Design review of the part built by this model. Coordinates are the model's own, in mm. Face numbers are marked on the shaded views. A direction names the side the tool comes from. Coordinates: 2 decimals unless noted, no trailing zeros. Write each loop counter-clockwise with the first axis right and the second up, starting at its lowest first coordinate (ties: lowest second). Pieces come first, ordered by that corner, then holes. Notation, with made-up numbers: (30, 1.25) - (74, 1.25) arc R12 cw to (74, 18.25) - close; hole circle Ø11 at (-37, 34.5). An arc over 180 degrees is marked (long way). Use a Markdown table: item, result.
Autodesk Inventor part; units mm, degrees
ref_plane "YZ Plane" through (0, 0, 0) normal (1, 0, 0) x (0, 1, 0)
ref_plane "XZ Plane" through (0, 0, 0) normal (0, 1, 0) x (-1, 0, 0)
ref_plane "XY Plane" through (0, 0, 0) normal (0, 0, 1) x (1, 0, 0)
sketch "Sketch2" plane through (0, 0, 0) normal (0, 0, 1) x (1, 0, 0)
  circle A0 centre (0, 0) radius 27.5
  circle A1 centre (0, 0) radius 8
  dimension "d0" = 55
  dimension "d1" = 16
extrude "Extrusion1" add sketch "Sketch2" along normal blind 6
sketch "Sketch3" plane through (0, 0, 6) normal (0, 0, 1) x (1, 0, 0)
  circle A0 centre (0, 0) radius 22.5 construction
  circle A1 centre (0, 0) radius 27.5
  line L0 (-5.87, 23.8) -> (-3.07, 23.8)
  line L1 (-3.07, 23.8) -> (-3.07, 16.8)
  line L2 (-3.07, 16.8) -> (-5.87, 16.8)
  line L3 (-5.87, 16.8) -> (-5.87, 23.8)
  line L4 (0, 0) -> (0, 27.8091) construction
  line L5 (3.07, 23.8) -> (5.87, 23.8)
  line L6 (5.87, 23.8) -> (5.87, 16.8)
  line L7 (5.87, 16.8) -> (3.07, 16.8)
  line L8 (3.07, 16.8) -> (3.07, 23.8)
  line L9 (-17.6764, -16.9836) -> (-19.0764, -14.5587)
  line L10 (-19.0764, -14.5587) -> (-13.0142, -11.0587)
  line L11 (-13.0142, -11.0587) -> (-11.6142, -13.4836)
  line L12 (-11.6142, -13.4836) -> (-17.6764, -16.9836)
  line L13 (-22.1464, -9.2413) -> (-23.5464, -6.8164)
  line L14 (-23.5464, -6.8164) -> (-17.4842, -3.3164)
  line L15 (-17.4842, -3.3164) -> (-16.0842, -5.7413)
  line L16 (-16.0842, -5.7413) -> (-22.1464, -9.2413)
  line L17 (23.5464, -6.8164) -> (22.1464, -9.2413)
  line L18 (22.1464, -9.2413) -> (16.0842, -5.7413)
  line L19 (16.0842, -5.7413) -> (17.4842, -3.3164)
  line L20 (17.4842, -3.3164) -> (23.5464, -6.8164)
  line L21 (19.0764, -14.5587) -> (17.6764, -16.9836)
  line L22 (17.6764, -16.9836) -> (11.6142, -13.4836)
  line L23 (11.6142, -13.4836) -> (13.0142, -11.0587)
  line L24 (13.0142, -11.0587) -> (19.0764, -14.5587)
  line L25 (0, 27.5) -> (22.8099, 27.5) construction
  circle A2 centre (0, 0) radius 27.5
  dimension "d4" = 5
  dimension "d5" = 2.8
  dimension "d6" = 7
  dimension "d9" = 2.8
  dimension "d10" = 7
  dimension "d12" = 3.07
  dimension "d13" = 3.07
  dimension "d16" = 360
  dimension "d20" = 3.7
extrude "Extrusion2" cut sketch "Sketch3" against normal blind 6 contours L0 L1 L2 L3 | L5 L6 L7 L8 | L9 L10 L11 L12 | L13 L14 L15 L16 | L17 L18 L19 L20 | L21 L22 L23 L24
sketch "Sketch7" plane through (0, 0, 6) normal (0, 0, 1) x (1, 0, 0)
  line L0 (19.5793, 23.0548) -> (11.3521, 18.3048)
  line L1 (11.3521, 18.3048) -> (8.3521, 23.501)
  line L2 (8.3521, 23.501) -> (16.5793, 28.251)
  line L3 (16.5793, 28.251) -> (19.5793, 23.0548)
  line L4 (23.5464, -6.8164) -> (5.87, 23.8) construction
  line L5 (5.87, 23.8) -> (16.4282, 29.8958) construction
  arc A0 (27.5, 0) -> (27.5, 0) centre (0, 0) ccw
  dimension "d16" = 360
  dimension "d59" = 6
  dimension "d60" = 9.5
  dimension "d100" = 2
  dimension "d101" = 1.5
extrude "Extrusion6" cut sketch "Sketch7" against normal blind 10 contours L0 A0 L2 L3 | L0 L1 L2 A0 picked at (10.9756, 21.9728)
sketch "Sketch6" plane through (0, 0, 6) normal (0, 0, 1) x (1, 0, 0)
  line L0 (23.5464, -6.8164) -> (5.87, 23.8) construction
  line L1 (-16.4532, 16.4649) -> (-19.4532, 21.6611)
  line L2 (-19.4532, 21.6611) -> (-14.2571, 24.6611)
  line L3 (-14.2571, 24.6611) -> (-11.2571, 19.4649)
  line L4 (-11.2571, 19.4649) -> (-16.4532, 16.4649)
  line L5 (-5.87, 16.8) -> (-5.87, 23.8)
  line L6 (-5.87, 23.8) -> (-7.957, 25.0049) construction
  line L7 (-23.5464, -6.8164) -> (-5.87, 23.8) construction
  circle A0 centre (0, 0) radius 27.5
  line L8 (10.8586, 11.6529) -> (13.2586, 7.496)
  circle A1 centre (0, 0) radius 8
  line L9 (5.87, 23.8) -> (-0.452, 20.15) construction
  line L10 (13.2586, 7.496) -> (0.9452, 0.3868)
  line L11 (10.8586, 11.6529) -> (-2.1318, 4.1529)
  line L12 (-2.1318, 4.1529) -> (0.9452, 0.3868)
  line L13 (17.0369, 21.5869) -> (11.3521, 18.3048)
  line L14 (11.3521, 18.3048) -> (8.3521, 23.501)
  dimension "d47" = 6
  dimension "d48" = 6
  dimension "d71" = 4.8
  dimension "d84" = 15.2302
  dimension "d96" = 14.2183
  dimension "d97" = 15
  dimension "d102" = 5.514
  dimension "d103" = 12.3093
  dimension "d104" = 19
extrude "Extrusion7" cut sketch "Sketch6" against normal blind 10 contours L1 A0 L3 L4 | L1 L2 L3 A0 | L8 L10 A1 L11 | A1 L10 L12 L11 picked at (-14.9352, 19.1568) picked at (0.7041, 3.9426)
fillet "Fillet4" radius 0.3 2 edges at (3.2988, 7.2882, 3) (6.996, 3.8802, 3)
sketch "Sketch13" plane through (0, 0, 6) normal (0, 0, 1) x (1, 0, 0)
  circle A0 centre (0, -18.0231) radius 6
  circle A1 centre (-17.6976, 6.6203) radius 5
  circle A2 centre (20.25, 3) radius 3.25
  circle A3 centre (17.6614, 12.6185) radius 2.5
  line L0 (-11.6142, -13.4836) -> (-17.6764, -16.9836)
  line L1 (17.6764, -16.9836) -> (11.6142, -13.4836)
  line L2 (-23.5464, -6.8164) -> (-17.4842, -3.3164)
  line L3 (-5.87, 16.8) -> (-5.87, 23.8)
  line L4 (-16.4532, 16.4649) -> (-18.6273, 20.2305)
  point P0 (0, 0)
  dimension "d146" = 12
  dimension "d147" = 6.5
  dimension "d148" = 10
  dimension "d151" = 5
  dimension "d154" = 9.7385
  dimension "d155" = 9.7385
  dimension "d156" = 8.7122
  dimension "d158" = 6
extrude "Extrusion16" cut sketch "Sketch13" against normal blind 10
properties part number "Gripper V 10.0 base 6mm"
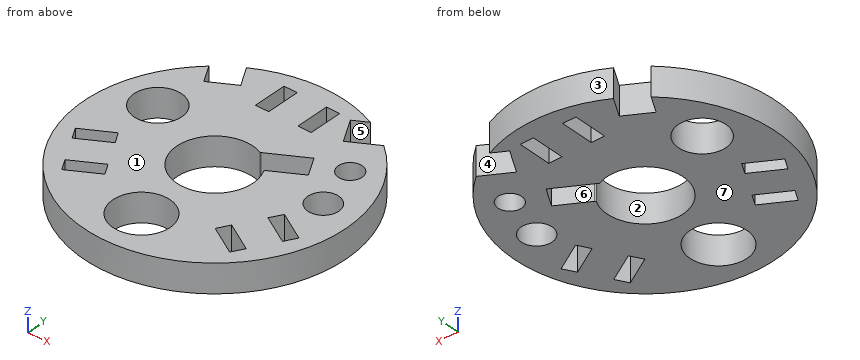
(1) Take a section at C-C on y = -22. Write out the cut boundary in (x, z), and give its area (3 significant figures).
Determined:
| item | result |
|---|---|
| outline | (-16.5, 0) - (-4.49, 0) - (-4.49, 6) - (-16.5, 6) - close; (4.49, 0) - (16.5, 0) - (16.5, 6) - (4.49, 6) - close |
| area | 144 mm2 |
(2) Take a section at D-D on z = 1.25. State how many separate pieces and enclosed holes the cut face has, and give its area (3 significant figures).
Determined:
| item | result |
|---|---|
| separate pieces | 1 |
| enclosed holes | 11 |
| area | 1,720 mm2 |
(3) Take a section at B-B on y = 3. Write out the cut boundary in (x, z), and give its area (3 significant figures).
Determined:
| item | result |
|---|---|
| outline | (-27.34, 0) - (-21.15, 0) - (-21.15, 6) - (-27.34, 6) - close; (-14.25, 0) - (-7.42, 0) - (-7.42, 6) - (-14.25, 6) - close; (7.42, 0) - (17, 0) - (17, 6) - (7.42, 6) - close; (23.5, 0) - (27.34, 0) - (27.34, 6) - (23.5, 6) - close |
| area | 159 mm2 |
(4) Take a section at A-A on x = 0. Write out the cut boundary in (y, z), and give its area (3 significant figures).
Determined:
| item | result |
|---|---|
| outline | (-27.5, 0) - (-24.02, 0) - (-24.02, 6) - (-27.5, 6) - close; (-12.02, 0) - (-8, 0) - (-8, 6) - (-12.02, 6) - close; (8, 0) - (27.5, 0) - (27.5, 6) - (8, 6) - close |
| area | 162 mm2 |
(5) For pin 1 (3 mm diameter, centred on y = 19, z = 2.5, fed in from -X); pin 2 (3 mm diameter, centred on y = 20, z = 2.5, fed in from +X); pin 3 (9.5 mm diameter, centred on x = 0, y = 0, fed in from +Z); pin 4 (1.8 mm diameter, centred on y = 20, z = 1.5, fed in from -X), all flat-tipped, find the tip position at first contact; note any pin that passes through.
Determined:
| item | result |
|---|---|
| pin 1 | x = -21.21 |
| pin 2 | x = 20.35 |
| pin 3 | through |
| pin 4 | x = -19.78 |
(6) Draft analysis for pull direction Y (two halves, no side actions). For the marked faces 1, 2 and 3, state which applies: +Y half, -Y half, draft (parallel to the pull), parting line (faces both ways), or undercut.
Determined:
| item | result |
|---|---|
| face 1 | draft |
| face 2 | undercut |
| face 3 | +Y half |
(7) Machinability: for the marked faces 4, 5, 6 and 7, which of the approach directions +Z, -Z, +X, -X, +Y, -Y give a long, thin tool a straight path to every point of the face, cutting with its end or side? Answer none if there is none.
Determined:
| item | result |
|---|---|
| face 4 | +Z, -Z, +Y |
| face 5 | +Z, -Z, +X |
| face 6 | +Z, -Z |
| face 7 | -Z, +X, -X, +Y, -Y |
(8) For L1, parallel to Y at x = 18, z = 1.7; L2, parallel to Y at x = 5.5, z = 4.35; L3, parallel to X at y = 9, z = 5.1, list the stretches that pass through material, from the lowest coordinate up. Write a range as from..to.
Determined:
| item | result |
|---|---|
| L1 | -20.79..-16.42, -13.94..-6.85, -3.61..0.65, 5.35..10.14, 15.1..20.79 |
| L2 | -26.94..-20.42, -15.63..-5.81, 8.56..16.8, 23.8..26.94 |
| L3 | -25.99..-22.09, -13.3..6.26, 12.39..25.99 |
